Job drawing, mm, ordinate dimensions from the low corner. One solid piece. Round coordinates to 2 decimals unless told otherwise and drop trailing zeros. Loops run counter-clockwise (first coordinate to the right, second up) from the corner with the lowest first, then second, coordinate; pieces in that order, holes last. Notation, with made-up numbers: M -12.75,-33 L 24.25,-33 A14 ccw 24.25,-14 Z; hole C 55.25,-3 d9. An arc over 180 degrees is marked long. Use one line per item in the form item = value. Start each with the question number.
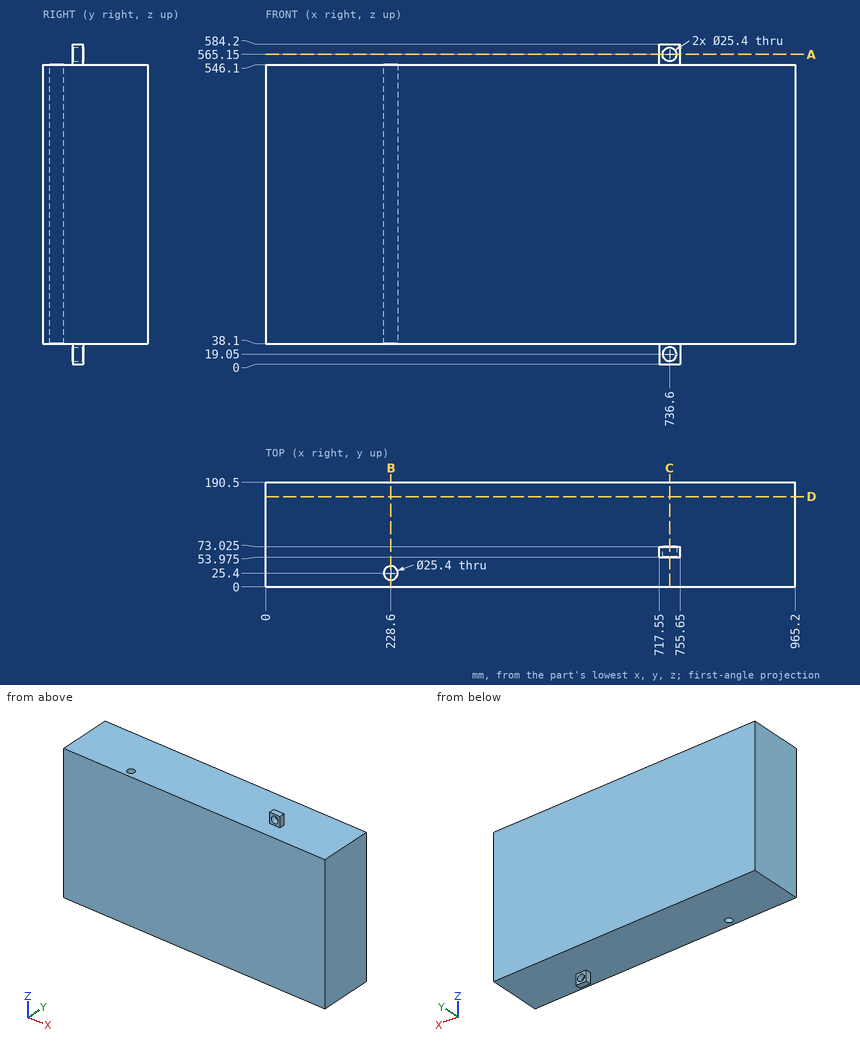
Q1. Wall check: probe 1 along Z at (x, y) = (736.6, 61.75); probe 2 along Y at (x, z) = (228.6, 368); probe 3 along Z at (x, y) = (683.5, 115). Give the ranges that are in metal, low to high.
Q2. Saw through at A-A (z = 565.15). Give the cut face in (x, y) (3 decimals).
Q3. Saw through at C-C (x = 736.6). Give the cut face in (y, z) (3 decimals), and give its area (3 significant figures).
Q4. Saw through at D-D (y = 164.5). Give the cut face in (x, z).
Q5. Drop flat-ended pins along their axis: P1, Ø15, axis at y = 59.5, z = 565.5, coming from the +X side; P2, Ø5, axis at x = 815.5, y = 99.5, coming from the +Z side; P3, Ø8, axis at x = 197.5, y = 73.5, coming from the -Z side; P4, Ø23, axis at x = 736.6, z = 565.15, coming from the +Y side. Give the stop position or say it passes through.
Q6. Saw through at B-B (x = 228.6). Give the cut face in (y, z).
Filled in:
q1.probe_1 = 0 to 6.35, 31.75 to 552.45, 577.85 to 584.2
q1.probe_2 = 0 to 12.7, 38.1 to 190.5
q1.probe_3 = 38.1 to 546.1
q2.outline = M 717.55,53.975 L 723.9,53.975 L 723.9,73.025 L 717.55,73.025 Z; M 749.3,53.975 L 755.65,53.975 L 755.65,73.025 L 749.3,73.025 Z
q3.outline = M 0,38.1 L 53.975,38.1 L 53.975,31.75 L 73.025,31.75 L 73.025,38.1 L 190.5,38.1 L 190.5,546.1 L 73.025,546.1 L 73.025,552.45 L 53.975,552.45 L 53.975,546.1 L 0,546.1 Z; M 53.975,0 L 73.025,0 L 73.025,6.35 L 53.975,6.35 Z; M 53.975,577.85 L 73.025,577.85 L 73.025,584.2 L 53.975,584.2 Z
q3.area = 97,300 mm²
q4.outline = M 0,38.1 L 965.2,38.1 L 965.2,546.1 L 0,546.1 Z
q5.P1 = 755.65
q5.P2 = 546.1
q5.P3 = 38.1
q5.P4 = through
q6.outline = M 0,38.1 L 12.7,38.1 L 12.7,546.1 L 0,546.1 Z; M 38.1,38.1 L 190.5,38.1 L 190.5,546.1 L 38.1,546.1 Z
